Part model, mm, in its own coordinate system. A direction names the side the tool comes from. Coordinates: 2 decimals unless noted, no trailing zeros. Order: outer loops, then holes, each group sorted by start corner. A loop starts at its lowest first (then second) coordinate and runs counter-clockwise, first axis right, second up.
```python
from build123d import *

# Parameters (mm, degrees)
F0_W     = 30
F0_H     = 30
F1_DEPTH = 300
F2_W     = 24
F2_H     = 24
F3_DEPTH = 300.001
F4_R     = 2.5
F5_DEPTH = 30.001


with BuildPart() as f1:
    # F0 (on Front) → F1 (new body)
    with BuildSketch(Plane.XZ):
        with Locations((15, 15)):
            Rectangle(F0_W, F0_H)
    extrude(amount=F1_DEPTH)

    # F2 (on face) → F3 (cut, through all)
    with BuildSketch(Plane.XZ.offset(300)):
        with Locations((15, 15)):
            Rectangle(F2_W, F2_H)
    extrude(amount=-F3_DEPTH, mode=Mode.SUBTRACT)

    # F4 (on face) → F5 (cut, through all)
    with BuildSketch(Plane.YZ.offset(30)):
        with Locations((-60, 14.536702)):
            Circle(F4_R)
    extrude(amount=-F5_DEPTH, mode=Mode.SUBTRACT)


solid = f1.part
```
(1) Slice it at A-A, the plane y = -60. Give the cut face in (x, z).
(2) Slice it at D-D, the plane y = -213.5. Give the cut face in (x, z), then the cut area to 3 significant figures.
(3) Tool access for faces 1 (the face through (15, -152, 3)), 2 (the face through (0, -148, 15)): list every direction of +Z, -Z, +X, -X, +Y, -Y with a clear straight run to the whole face (end or side of a thin tool).
(4) Probe line 1 (Z direction, x = 24, y = -91.5); line 2 (Z direction, x = 1.65, y = -60). List the from-to ranges inside material, lowest first.
(5) Slice it at B-B, the plane z = 23.5. Give the cut face in (x, y), then the cut area to 3 significant figures.
(6) Pull direction Y, two halves, no side cores. Call faces 3 (the face through (30, -148, 15)), 4 (the face through (28, 0, 15)), 5 (the face through (28, -300, 15)), 6 (the face through (1.521, -57.615, 15.288)): +Y half, -Y half, draft (parallel to the pull), parting line (faces both ways), or undercut.
(7) Slice it at C-C, the plane x = 21.5. Give the cut face in (y, z).
(8) Drop a flat-ended pin along its axis: pin 1 (10 mm diameter, centred on x = 9.5, z = 18, fed in from +Y). Give the stop position or say it passes through.
Here are the results:
1. outline: (0, 0) - (30, 0) - (30, 12.04) - (27, 12.04) - (27, 3) - (3, 3) - (3, 12.04) - (0, 12.04) - close; (0, 17.04) - (3, 17.04) - (3, 27) - (27, 27) - (27, 17.04) - (30, 17.04) - (30, 30) - (0, 30) - close
2. outline: (0, 0) - (30, 0) - (30, 30) - (0, 30) - close; hole (3, 3) - (27, 3) - (27, 27) - (3, 27) - close
2. area: 324 mm2
3. face 1: +Y, -Y
3. face 2: +Z, -Z, -X, +Y, -Y
4. line 1: z = 0 to 3, 27 to 30
4. line 2: z = 0 to 12.04, 17.04 to 30
5. outline: (0, -300) - (3, -300) - (3, 0) - (0, 0) - close; (27, -300) - (30, -300) - (30, 0) - (27, 0) - close
5. area: 1,800 mm2
6. face 3: draft
6. face 4: +Y half
6. face 5: -Y half
6. face 6: undercut
7. outline: (-300, 0) - (0, 0) - (0, 3) - (-300, 3) - close; (-300, 27) - (0, 27) - (0, 30) - (-300, 30) - close
8. pin 1: passes through
